```python
from build123d import *

# Parameters (mm, degrees)
SKETCH1_RX               = 150
SKETCH1_RY               = 100
BOSS_EXTRUDE1_DEPTH      = 5
CUT_EXTRUDE1_DEPTH       = 181.346887969
CUT_EXTRUDE2_DEPTH       = 181.346887969
CUT_EXTRUDE3_DEPTH       = 181.346887969
CUT_EXTRUDE4_DEPTH       = 181.346887969
CUT_EXTRUDE5_DEPTH       = 181.346887969
SKETCH11_W               = 1.375
SKETCH11_H               = 12.5
SKETCH12_W               = 1.375
SKETCH12_H               = 12.5
SKETCH13_W               = 1.375
SKETCH13_H               = 12.5
SKETCH14_W               = 1.375
SKETCH14_H               = 12.5
F_3_0_3_DIAMETER_HOLE1_D = 3


with BuildPart() as part:
    # Sketch1 → Boss-Extrude1 (new body)
    with BuildSketch(Plane.XY.offset(5)):
        with Locations(Location((0, 0), (0, 0, 0))):
            Ellipse(SKETCH1_RX, SKETCH1_RY)
    extrude(amount=-BOSS_EXTRUDE1_DEPTH)

    # Sketch2 → Cut-Extrude1 (cut, through all)
    with BuildSketch(Plane(origin=(0, 0, 0), x_dir=(-1, 0, 0), z_dir=(0, 0, -1))):
        with BuildLine():
            Line((25.9, 24.5), (-25.9, 24.5))
            ThreePointArc((-25.9, 24.5), (-26.807968978, 22.307968978), (-29, 21.4))
            Line((-29, 21.4), (-29, -21.4))
            ThreePointArc((-29, -21.4), (-26.807968978, -22.307968978), (-25.9, -24.5))
            Line((-25.9, -24.5), (25.9, -24.5))
            ThreePointArc((25.9, -24.5), (26.807968978, -22.307968978), (29, -21.4))
            Line((29, -21.4), (29, 21.4))
            ThreePointArc((29, 21.4), (26.807968978, 22.307968978), (25.9, 24.5))
        make_face()
    extrude(amount=-CUT_EXTRUDE1_DEPTH, mode=Mode.SUBTRACT)

    # Sketch7 → Cut-Extrude2 (cut, through all)
    with BuildSketch(Plane.XY.offset(5)):
        Polygon((45.191487885, -51.097974081), (76.599310052, -77.452266078), (89.197947202, -62.437794993), (57.790125034, -36.083502996), align=None)
    extrude(amount=-CUT_EXTRUDE2_DEPTH, mode=Mode.SUBTRACT)

    # Sketch8 → Cut-Extrude3 (cut, through all)
    with BuildSketch(Plane.XY.offset(5)):
        Polygon((-76.598710341, -77.451785496), (-45.190888173, -51.097493499), (-57.789525323, -36.083022414), (-89.197347491, -62.437314411), align=None)
    extrude(amount=-CUT_EXTRUDE3_DEPTH, mode=Mode.SUBTRACT)

    # Sketch9 → Cut-Extrude4 (cut, through all)
    with BuildSketch(Plane.XY.offset(5)):
        Polygon((-45.191671729, 51.098342778), (-76.599493897, 77.452634775), (-89.198131047, 62.43816369), (-57.790308879, 36.083871693), align=None)
    extrude(amount=-CUT_EXTRUDE4_DEPTH, mode=Mode.SUBTRACT)

    # Sketch10 → Cut-Extrude5 (cut, through all)
    with BuildSketch(Plane(origin=(0, 0, 0), x_dir=(-1, 0, 0), z_dir=(0, 0, -1))):
        Polygon((-89.198042922, 62.437370539), (-57.790220755, 36.083078542), (-45.191583605, 51.097549627), (-76.599405773, 77.451841624), align=None)
    extrude(amount=-CUT_EXTRUDE5_DEPTH, mode=Mode.SUBTRACT)

    # Sketch11 → Cut-Revolve1 (revolve, cut)
    with BuildSketch(Plane(origin=(0, -24.5, 0), x_dir=(1, 0, 0), z_dir=(0, 1, 0))):
        with Locations((29.6875, -6.25)):
            Rectangle(SKETCH11_W, SKETCH11_H)
    revolve(axis=Axis((29, -24.5, 0), (0, 0, 1)), mode=Mode.SUBTRACT)

    # Sketch12 → Cut-Revolve2 (revolve, cut)
    with BuildSketch(Plane(origin=(0, 24.5, 0), x_dir=(1, 0, 0), z_dir=(0, 1, 0))):
        with Locations((29.6875, -6.25)):
            Rectangle(SKETCH12_W, SKETCH12_H)
    revolve(axis=Axis((29, 24.5, 0), (0, 0, 1)), mode=Mode.SUBTRACT)

    # Sketch13 → Cut-Revolve3 (revolve, cut)
    with BuildSketch(Plane(origin=(0, 24.5, 0), x_dir=(1, 0, 0), z_dir=(0, 1, 0))):
        with Locations((-28.3125, -6.25)):
            Rectangle(SKETCH13_W, SKETCH13_H)
    revolve(axis=Axis((-29, 24.5, 0), (0, 0, 1)), mode=Mode.SUBTRACT)

    # Sketch14 → Cut-Revolve4 (revolve, cut)
    with BuildSketch(Plane(origin=(0, -24.5, 0), x_dir=(1, 0, 0), z_dir=(0, 1, 0))):
        with Locations((-28.3125, -6.25)):
            Rectangle(SKETCH14_W, SKETCH14_H)
    revolve(axis=Axis((-29, -24.5, 0), (0, 0, 1)), mode=Mode.SUBTRACT)

    # Ø3.0 (3) Diameter Hole1 (through all)
    with Locations(Plane.XY.offset(5)):
        with Locations((82.454776258, -76.230171352), (89.011209876, -68.416518032), (45.378225211, -45.119251043), (-45.378409055, 45.119619739), (-45.377625499, -45.118770461), (-51.934059118, -37.305117141), (-82.454176546, -76.22969077), (-89.010610165, -68.41603745), (51.934658829, -37.305597723), (51.93475455, 37.305173269), (45.378320931, 45.118826588), (82.454871978, 76.229746897), (-51.934842674, 37.305966419), (-82.454960102, 76.230540048), (-89.011393721, 68.416886728), (89.011305596, 68.416093578)):
            Hole(F_3_0_3_DIAMETER_HOLE1_D / 2)


solid = part.part
```
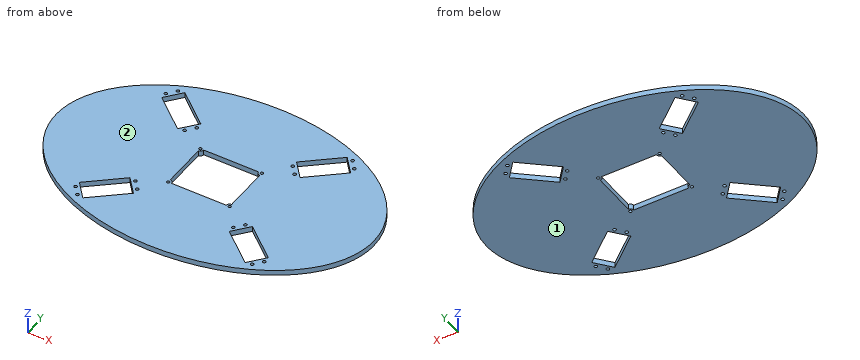
Input: part model. Units: mm. Frame: model coordinates. Face numbers are marked on the shaded views. Round coordinates to 2 decimals unless told otherwise and drop trailing zeros. One line per item, written item: value. Start each with the question number.
(1) Section A-A, the plane z = 0.75. Count the separate pieces of the cut face and the enclosed holes in it, plus the area to 3 significant figures.
(2) Draft query along Z for the marked faces 1 and 2. Return one class per face: +Z half, -Z half, draft (parallel to the pull), parting line (faces both ways), or undercut.
(3) Contact query for flat-ended pins moving along their axis: P1, Ø2.5, axis at x = -8, z = 3.5, coming from the +Y side; P2, Ø3, axis at x = 8.5, z = 2.5, coming from the -Y side; P3, Ø1, axis at y = 38.5, z = 1.5, coming from the -X side. Output: stop coordinate, or through.
(4) Ray query, line 1 (X direction, y = -42, z = 3.75); line 2 (X direction, y = 52, z = 1.8); line 3 (X direction, y = -76, z = 1.25). Return the intervals inside material, ascending. Write a range as [from, to].
Results below:
1. separate pieces: 1
1. enclosed holes: 25
1. area: 41,000 mm^2
2. face 1: -Z half
2. face 2: +Z half
3. P1: y = 99.9
3. P2: y = -99.89
3. P3: x = -138.75
4. line 1: [-136.13, -64.84], [-52.82, 52.83], [64.84, 136.13]
4. line 2: [-128.12, -76.76], [-46.27, 46.27], [76.76, 128.12]
4. line 3: [-97.49, -83.94], [-80.97, -77.82], [-74.87, 74.87], [77.82, 80.97], [83.94, 97.49]
